Input: part model. Units: mm. Frame: model coordinates. A direction names the side the tool comes from. Round coordinates to 2 decimals unless told otherwise and drop trailing zeros. Loops run counter-clockwise (first coordinate to the right, second up) from the corner with the lowest first, then second, coordinate; pieces in that order, holes last. Notation, with made-up numbers: M 89,86 L 133,86 A15 ccw 133,112 Z; hole C 52.5,62.25 d5. An arc over 180 degrees is marked long. Put each result on its own line as item: value. Start each with the question number.
1) Section B-B on x = -9.5. Output: boundary loops of the cut face in (y, z) (3 decimals), plus the area to 3 significant figures.
2) Pin query (flat end, axial travel): pin 1 (6 mm diameter, centred on x = -1.5, y = 1.5, fed in from +Z); pin 2 (1.5 mm diameter, centred on x = -5.5, y = -48.5, fed in from +Z); pin 3 (0.7 mm diameter, centred on x = 0.5, z = -1.5, fed in from -Y); pin 4 (2 mm diameter, centred on y = 1, z = 7.5, fed in from -X). Return the tip coordinate at first contact, or that it passes through.
3) Section C-C on z = 6.75. Output: boundary loops of the cut face in (x, y), plus the area to 3 significant figures.
4) Section D-D on y = -28. Output: boundary loops of the cut face in (x, z).
5) Draft query along Z for faces 1 (the face through (3, 3, 10.414)), 2 (the face through (0.229, -36.356, 0.378)), 3 (the face through (0, 6, 0.635)), 4 (the face through (-1.06, 4.773, 6.619)). Return one class per face: +Z half, -Z half, draft (parallel to the pull), parting line (faces both ways), or undercut.
6) Section A-A on y = -38.1. Output: boundary loops of the cut face in (x, z).
7) Reachability of faces 5 (the face through (0, -51, -0.254)), 6 (the face through (16.192, -23, 2)), 7 (the face through (-1.404, 6.323, 9.121)) from +Z, -Z, +X, -X, +Y, -Y: full face, straight path, thin tool, end or side. Return the list, or none.
8) Line query: probe 1 along Y at (x, z) = (0, 1.4); probe 2 along Y at (x, z) = (0, -0.05); probe 3 along X at (y, z) = (-13.97, -1). Output: solid intervals per line, ascending.
from build123d import *

# Parameters (mm, degrees)
F2_R            = 0.508
F3_S5_R         = 4.8895
F3_T6_DEPTH     = 11
F4_R            = 0.254
F5_W            = 70.612
F5_H            = 7.62
F6_DEPTH        = 16.1925
F7_W            = 14.224
F7_H            = 3.175
F7_H_2          = 2.286
F8_DEPTH        = 32.386
F10_D           = 3.5179
F10_CSINK_D     = 6.477
F10_CSINK_ANGLE = 82


# Not quite as in the source:
# - a fillet or chamfer that OpenCascade refuses, or shapes differently, is made with other operations: its cross-section is extruded or revolved along the edge and cut away or added


with BuildPart() as f1:
    # F0 (on Front) → F1 (revolve)
    with BuildSketch(Plane.XZ):
        Polygon((0, 9.271), (0, 0), (11.1125, 0), (11.1125, 5.08), (4.8895, 5.08), (4.8895, 7.62), (6.477, 7.62), (6.477, 10.414), (3.6195, 10.414), (3.6195, 9.271), align=None)
    revolve(axis=Axis((0, 0, 5.207), (0, 0, -1)))

    # F2
    f2_edges = [f1.edges().sort_by_distance(p)[0] for p in [
        (-6.477, 0, 10.414),
        (-4.8895, 0, 5.08),
    ]]
    fillet(f2_edges, radius=F2_R)

    # F3: chamfer of 0.508 x 1.5917743649 on 1 edges, made by hand


with BuildPart() as f3_tool2:
    # F3_s3 → F3_t4 (revolve)
    with BuildSketch(Plane.XZ):
        Polygon((4.8852256351, 7.62), (6.477, 8.128), (6.477, 7.62), align=None)
    revolve(axis=Axis((0, 0, 7.62), (0, 0, -1)))

    # F3_s5 → F3_t6 (cut, symmetric)
    with BuildSketch(Plane.XY.offset(7.9)):
        Circle(F3_S5_R)
    extrude(amount=F3_T6_DEPTH, both=True, mode=Mode.SUBTRACT)


with BuildPart() as f1_1:
    add(f1.part)

    # F3_t1: cut F3_tool2
    add(f3_tool2.part, mode=Mode.SUBTRACT)

    # F4
    f4_edges = [f1_1.edges().sort_by_distance(p)[0] for p in [
        (-6.477, 0, 8.128),
    ]]
    fillet(f4_edges, radius=F4_R)

    # F5 (on Right) → F6 (join, symmetric)
    with BuildSketch(Plane.YZ):
        with Locations((-22.606, 1.27)):
            Rectangle(F5_W, F5_H)
    extrude(amount=F6_DEPTH, both=True)

    # F7 (on face) → F8 (cut, through all)
    with BuildSketch(Plane(origin=(-16.1925, 0, 0), x_dir=(0, -1, 0), z_dir=(-1, 0, 0))):
        with Locations((-5.588, -0.9525)):
            Rectangle(F7_W, F7_H)
        with Locations((50.8, -1.397)):
            Rectangle(F7_W, F7_H_2)
    extrude(amount=-F8_DEPTH, mode=Mode.SUBTRACT)

    # F10 (through all)
    with Locations(Plane.XY.offset(5.08)):
        with Locations((0, -13.97), (0, -38.1)):
            CounterSinkHole(F10_D / 2, F10_CSINK_D / 2, counter_sink_angle=F10_CSINK_ANGLE)


solid = f1_1.part
Geometry results:
1. outline: M -57.912,-0.254 L -43.688,-0.254 L -43.688,-2.54 L -1.524,-2.54 L -1.524,0.635 L 12.7,0.635 L 12.7,5.08 L -57.912,5.08 Z
1. area: 460 mm²
2. pin 1: stops at z = 10.41
2. pin 2: stops at z = 5.08
2. pin 3: stops at y = -43.69
2. pin 4: stops at x = -6.46
3. outline: C 0,0 d9.78
3. area: 75.1 mm²
4. outline: M -16.19,-2.54 L 16.19,-2.54 L 16.19,5.08 L -16.19,5.08 Z
5. face 1: +Z half
5. face 2: draft
5. face 3: -Z half
5. face 4: undercut
6. outline: M -16.19,-2.54 L -1.76,-2.54 L -1.76,3.38 L -3.24,5.08 L -16.19,5.08 Z; M 1.76,-2.54 L 16.19,-2.54 L 16.19,5.08 L 3.24,5.08 L 1.76,3.38 Z
7. face 5: -Z, +X, -X, -Y
7. face 6: +Z, -Z, +X, +Y, -Y
7. face 7: +Z
8. probe 1: y = -57.91 to -39.86, -36.34 to -15.73, -12.21 to 12.7
8. probe 2: y = -57.91 to -39.86, -36.34 to -15.73, -12.21 to -1.52
8. probe 3: x = -16.19 to -1.76, 1.76 to 16.19
